Read the model definition and answer for the solid it produces. Units are mm, in the model's axes. A direction names the side the tool comes from. Coordinates: 2 decimals unless noted, no trailing zeros. Loops run counter-clockwise (first coordinate to the right, second up) from the corner with the lowest first, then second, coordinate; pieces in that order, holes last. Notation, with made-up numbers: (-31, 36.25) - (1, 36.25) arc R26 ccw to (1, 51.25) - close; hole circle Ø4 at (-14, -30.75). An arc over 180 degrees is marked (long way). Use one line per item in the form item = value. Start each with the question number.
1) A cutting plane is placed at C-C (y = -5). Give the vertices of the cut face in (x, z), and give its area (3 significant figures).
2) Each of these flat-tipped pins is pushed along its axis until it touches: P1, Ø8, axis at x = 14.5, y = -12, coming from the +Z side; P2, Ø5, axis at x = 14.5, y = -8, coming from the +Z side; P3, Ø10, axis at y = -10.5, z = 5.5, coming from the +X side (3 decimals). Where does it stop, or does it pass through?
3) The mould has two halves that part along X. Classify faces 3 (the face through (23.846, -10.353, 7.509)), 4 (the face through (-14.985, -20.986, 0.66)), 5 (the face through (0, -22, -16)): released by +X, released by -X, zero draft, split by the parting line, or undercut.
4) A cutting plane is placed at B-B (z = 0). Give the vertices of the cut face in (x, y), and give its area (3 significant figures).
5) A cutting plane is placed at A-A (x = 0). Give the vertices of the cut face in (y, z), and give its area (3 significant figures).
6) Consider line 1 (Z direction, x = 0, y = -8.25); line 2 (Y direction, x = -9, z = -13); line 3 (Z direction, x = -20, y = -10.25). Determine where each line is inside the solid, lowest interval first.
7) Which of the six approach directions +Z, -Z, +X, -X, +Y, -Y give full straight-line access (tool end or side, diameter ignored) to faces 1 (the face through (-17, 0, -5)), 2 (the face through (13, -20, 8))?
from build123d import *

# Parameters (mm, degrees)
F0_R     = 25
F0_R_2   = 17.5
F1_DEPTH = 20
F2_R     = 25
F2_R_2   = 15
F3_DEPTH = 2
F4_SIZE  = 1


with BuildPart() as f1:
    # F0 (on Front) → F1 (new body)
    with BuildSketch(Plane.XZ):
        Circle(F0_R)
        Circle(F0_R_2, mode=Mode.SUBTRACT)
    extrude(amount=F1_DEPTH)

    # F2 (on face) → F3 (join)
    with BuildSketch(Plane.XZ.offset(20)):
        Circle(F2_R)
        Circle(F2_R_2, mode=Mode.SUBTRACT)
    extrude(amount=F3_DEPTH)

    # F4
    f4_edges = [f1.edges().sort_by_distance(p)[0] for p in [
        (-25, -22, 0),
    ]]
    chamfer(f4_edges, length=F4_SIZE)


solid = f1.part
Found:
q1.outline = circle Ø50 at (0, 0); hole circle Ø35 at (0, 0)
q1.area = 1,000 mm^2
q2.P1 = 22.69
q2.P2 = 21.93
q2.P3 = 24.995
q3.face_3 = split by the parting line
q3.face_4 = undercut
q3.face_5 = zero draft
q4.outline = (-25, -21) - (-24, -22) - (-15, -22) - (-15, -20) - (-17.5, -20) - (-17.5, 0) - (-25, 0) - close; (15, -22) - (24, -22) - (25, -21) - (25, 0) - (17.5, 0) - (17.5, -20) - (15, -20) - close
q4.area = 339 mm^2
q5.outline = (-22, -24) - (-21, -25) - (0, -25) - (0, -17.5) - (-20, -17.5) - (-20, -15) - (-22, -15) - close; (-22, 15) - (-20, 15) - (-20, 17.5) - (0, 17.5) - (0, 25) - (-21, 25) - (-22, 24) - close
q5.area = 339 mm^2
q6.line_1 = -25 to -17.5, 17.5 to 25
q6.line_2 = -22 to -20
q6.line_3 = -15 to 15
q7.face_1 = +Z, -Z, +X, -X, +Y
q7.face_2 = +Y
